Input: dimensioned drawing with shaded views. Units: mm. Origin: part minimum x, y, z. A direction names the side the tool comes from. Round coordinates to 2 decimals unless told otherwise and drop trailing zeros. Loops run counter-clockwise (first coordinate to the right, second up) from the corner with the lowest first, then second, coordinate; pieces in that order, holes last. Notation, with made-up numbers: (-24, 32) - (24, 32) arc R33 ccw to (24, 62) - close; hole circle Ø9 at (-12.5, -13). An arc over 180 degrees is marked (long way). Answer as CSV lines item,"result".
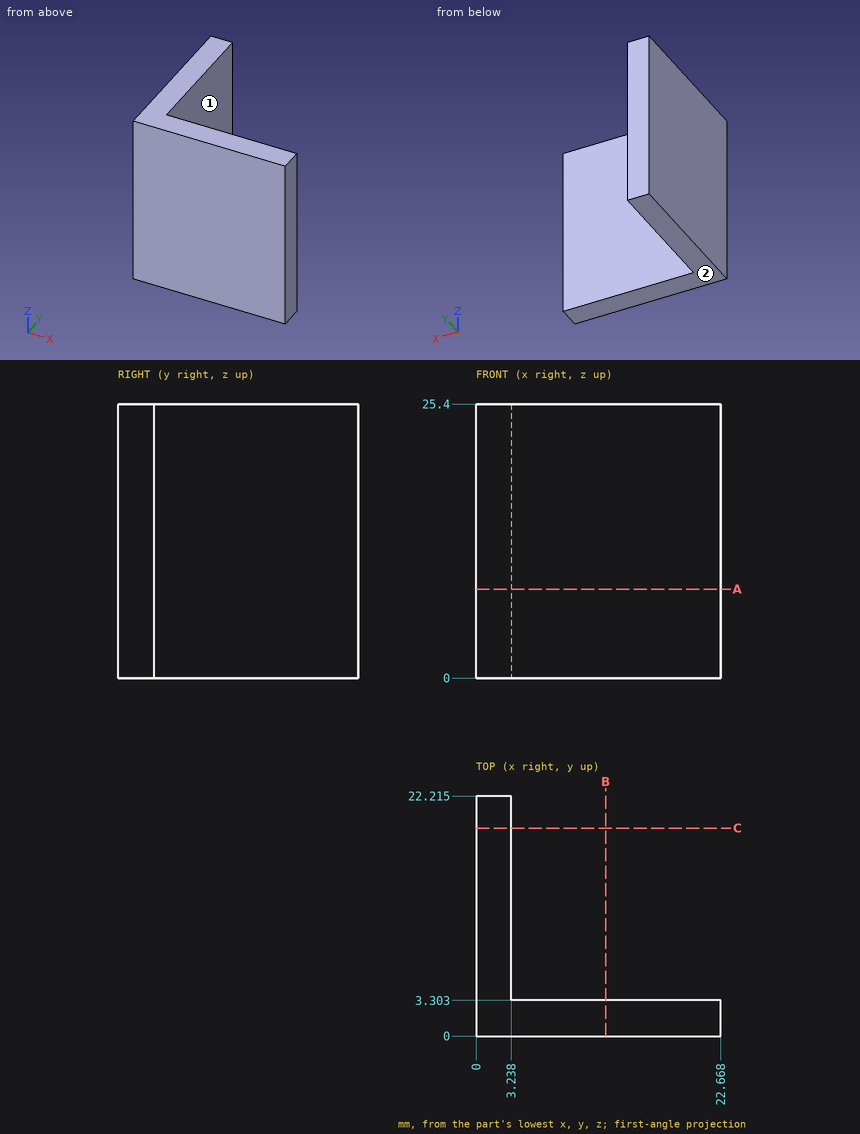
(1) Section B-B (x = 12). Output: boundary loops of the cut face in (y, z).
Findings below:
outline,"(0, 0) - (3.3, 0) - (3.3, 25.4) - (0, 25.4) - close"
(2) Pin query (flat end, axial travel): P1, Ø5, axis at x = 9, z = 4.5, coming from the +Y side; P2, Ø10, axis at y = 9.5, z = 18.5, coming from the +X side. Return the tip coordinate at first contact, or that it passes through.
Findings below:
P1,"y = 3.3"
P2,"x = 3.24"
(3) Material intervals for line 1 along X through (y, z) = (16, 12); line 2 along Y through (x, z) = (13.75, 20.5), sorted ascending.
Findings below:
line 1,"0 to 3.24"
line 2,"0 to 3.3"
(4) Section A-A (z = 8.25). Output: boundary loops of the cut face in (x, y) (1 decimal).
Findings below:
outline,"(0, 0) - (22.7, 0) - (22.7, 3.3) - (3.2, 3.3) - (3.2, 22.2) - (0, 22.2) - close"
(5) Section C-C (y = 19.25). Output: boundary loops of the cut face in (x, z).
Findings below:
outline,"(0, 0) - (3.24, 0) - (3.24, 25.4) - (0, 25.4) - close"
(6) Access query for the marked faces 1 and 2. Directions: +Z, -Z, +X, -X, +Y, -Y. A direction counts if a zero-diameter tool reaches every point of the face in a straight line with its end or side. Return the directions, or none.
Findings below:
face 1,"+Z, -Z, +X, +Y"
face 2,"-Z, +X, -X, +Y, -Y"
